The listing builds one solid part. Answer for the finished solid, in the listing's coordinates (mm). A direction names the side the tool comes from. Coordinates: 2 decimals unless noted, no trailing zeros.
from build123d import *

# Parameters (mm, degrees)
F0_W     = 25.4
F0_H     = 63.5
F1_DEPTH = 25.4
F3_DEPTH = 25.4
F5_DEPTH = 25.4
F7_DEPTH = 25.4
F8_R     = 2.54


with BuildPart() as f1:
    # F0 (on Front) → F1 (new body)
    with BuildSketch(Plane.XZ):
        with Locations((-12.7, 31.75)):
            Rectangle(F0_W, F0_H)
    extrude(amount=F1_DEPTH)

    # F2 (on face) → F3 (cut)
    with BuildSketch(Plane.XZ.offset(25.4)):
        with BuildLine():
            Line((-16.826138, 0), (-16.826138, 43.294895))
            ThreePointArc((-16.826138, 43.294895), (-15.979296, 57.029675), (-4.20577, 49.906094))
            ThreePointArc((-4.20577, 49.906094), (-5.124016, 46.174395), (-7.669056, 43.294895))
            Line((-7.669056, 43.294895), (-7.669056, 0))
            Line((-7.669056, 0), (0, 0))
            Line((0, 0), (0, 63.5))
            Line((0, 63.5), (-25.4, 63.5))
            Line((-25.4, 63.5), (-25.4, 0))
            Line((-25.4, 0), (-16.826138, 0))
        make_face()
    extrude(amount=-F3_DEPTH, mode=Mode.SUBTRACT)

    # F4 (on Right) → F5 (cut)
    with BuildSketch(Plane.YZ):
        Polygon((5.837639, 43.267213), (-8.126909, 43.267213), (-8.355836, -3.662833), (5.837639, -3.662833), align=None)
    extrude(amount=-F5_DEPTH, mode=Mode.SUBTRACT)

    # F6 (on Right) → F7 (cut)
    with BuildSketch(Plane.YZ):
        Polygon((-16.368283, -6.409957), (-15.91043, 43.267213), (-32.622103, 43.267213), (-32.622103, -6.409957), align=None)
    extrude(amount=-F7_DEPTH, mode=Mode.SUBTRACT)

    # F8
    f8_edges = [f1.edges().sort_by_distance(p)[0] for p in [
        (-16.826138, -8.232439, 21.633606),
        (-16.826138, -16.109818, 21.633606),
        (-7.669056, -16.109818, 21.633606),
        (-7.669056, -8.232439, 21.633606),
        (-15.979296, -25.4, 57.029675),
        (-15.979296, 0, 57.029675),
    ]]
    fillet(f8_edges, radius=F8_R)


solid = f1.part
1. Find the intervals of material crossed by L1, parallel to X at y = -10.5, z = 35.5; L2, parallel to Z at x = -18.75, y = -2; L3, parallel to Z at x = -15, y = -3, in increasing order.
Results found:
L1: x = -16.82 to -7.68
L2: z = 45.27 to 54.54
L3: z = 43.27 to 57.46
2. Flat-ended cylindrical pins translate along their axes: P1, Ø7.5, axis at x = -11.5, y = -20, coming from the -Z side; P2, Ø1, axis at x = -9.5, y = -18.5, coming from the +Z side; P3, Ø3, axis at x = -18.5, z = 38, coming from the +Y side; P4, Ø10, axis at y = -4.5, z = 14, coming from the +X side. Find the tip coordinate at first contact, or state that the pin passes through.
Results found:
P1: stops at z = 0
P2: stops at z = 57.63
P3: passes through
P4: stops at x = -8.03
3. A tool of negligible diameter and unlimited length cuts with its end or side. For faces 1 (the cylindrical face through (-16.062, -15.383, 21.942)), 2 (the cylindrical face through (-16.062, -8.958, 21.328)), 3 (the cylindrical face through (-8.393, -15.349, 21.335)), 4 (the cylindrical face through (-8.43, -8.96, 21.93)), from which of +Z, -Z, +X, -X, +Y, -Y can it reach the whole face along a straight path? Write none if from no direction.
Results found:
face 1: -X, -Y
face 2: -Z, -X, +Y
face 3: +X, -Y
face 4: -Z, +X, +Y
